Check sheet for the modelled part. Datum: model origin and axes. Units: mm. Face numbers are marked on the shaded views. A direction names the side the tool comes from. Coordinates: 2 decimals unless noted, no trailing zeros. Order: outer loops, then holes, each group sorted by start corner. A loop starts at its lowest first (then second) coordinate and runs counter-clockwise, first axis right, second up. Notation, with made-up numbers: M -1,-20 L 55,-20 A18 ccw 55,-1 Z; hole C -12,28 d8. An arc over 180 degrees is marked long. Answer in a Markdown table with one row per item. Add a question column.
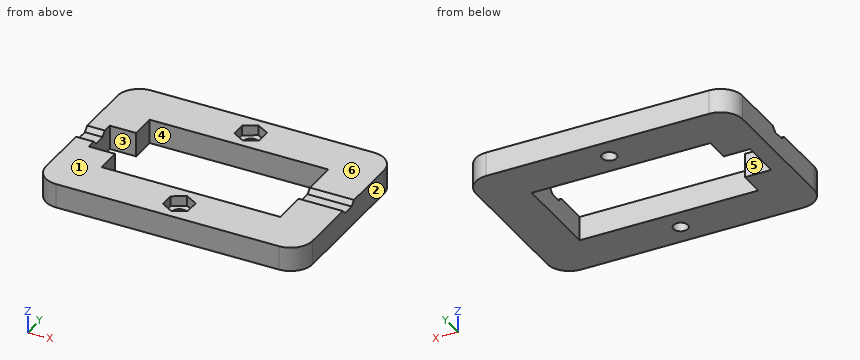
from build123d import *

# Parameters (mm, degrees)
F0_W     = 60.5
F0_H     = 40.5
F0_W_2   = 40.5
F0_H_2   = 20.5
F1_DEPTH = 5.5
F2_W     = 10
F2_H     = 2.8
F3_DEPTH = 1
F4_R     = 1.65
F5_DEPTH = 25
F6_W     = 6
F6_H     = 9
F7_DEPTH = 25
F9_DEPTH = 2.3
F10_SIZE = 0.99999
F11_R    = 5


# Not quite as in the source:
# - a fillet or chamfer is up to 0.001 mm smaller than in the source, because OpenCascade refuses the exact size


with BuildPart() as f1:
    # F0 (on Top) → F1 (new body)
    with BuildSketch(Plane.XY):
        Rectangle(F0_W, F0_H)
        Rectangle(F0_W_2, F0_H_2, mode=Mode.SUBTRACT)
    extrude(amount=F1_DEPTH)

    # F2 (on face) → F3 (cut)
    with BuildSketch(Plane.XY.offset(5.5)):
        with Locations((-25.25, 0)):
            Rectangle(F2_W, F2_H)
        with Locations((25.25, 0)):
            Rectangle(F2_W, F2_H)
    extrude(amount=-F3_DEPTH, mode=Mode.SUBTRACT)

    # F4 (on face) → F5 (cut)
    with BuildSketch(Plane.XY.offset(5.5)):
        with Locations((0, 15.25)):
            Circle(F4_R)
        with Locations((0, -15.25)):
            Circle(F4_R)
    extrude(amount=-F5_DEPTH, mode=Mode.SUBTRACT)

    # F6 (on face) → F7 (cut)
    with BuildSketch(Plane(origin=(0, 0, 0), x_dir=(1, 0, 0), z_dir=(0, 0, -1))):
        with Locations((-23.25, 0)):
            Rectangle(F6_W, F6_H)
    extrude(amount=-F7_DEPTH, mode=Mode.SUBTRACT)

    # F8 (on face) → F9 (cut)
    with BuildSketch(Plane.XY.offset(5.5)):
        Polygon((2.85, 13.6045517328), (2.85, 16.8954482672), (0, 18.5408965344), (-2.85, 16.8954482672), (-2.85, 13.6045517328), (0, 11.9591034656), align=None)
        Polygon((-2.85, -16.8954482672), (0, -18.5408965344), (2.85, -16.8954482672), (2.85, -13.6045517328), (0, -11.9591034656), (-2.85, -13.6045517328), align=None)
    extrude(amount=-F9_DEPTH, mode=Mode.SUBTRACT)

    # F10 (size 1 in the source; OpenCascade refuses exactly that, so slightly less here)
    f10_edges = [f1.edges().sort_by_distance(p)[0] for p in [
        (25.25, 1.4, 5.5),
        (25.25, -1.4, 5.5),
        (-28.25, 1.4, 5.5),
        (-28.25, -1.4, 5.5),
    ]]
    chamfer(f10_edges, length=F10_SIZE)

    # F11
    f11_edges = [f1.edges().sort_by_distance(p)[0] for p in [
        (30.25, 20.25, 2.75),
        (30.25, -20.25, 2.75),
        (-30.25, -20.25, 2.75),
        (-30.25, 20.25, 2.75),
    ]]
    fillet(f11_edges, radius=F11_R)


solid = f1.part
1. Section check A-A on x = 17. Enter the section's corners in (y, z), then the cut area to 3 significant figures.
2. Set-up check for the marked faces 5 and 6: record each of +Z, -Z, +X, -X, +Y, -Y from which the full face is reachable in a straight line by a thin tool's end or side.
3. Scan lines: line 1 (Y direction, x = 0, z = 0.85); line 2 (Y direction, x = -8, z = 3.9); line 3 (X direction, y = -7, z = 4.05). Record each from-to range of solid material in increasing order.
4. Go/stop test with flat-tipped pins: pin 1 Ø0.8 at (x, y) = (25.5, 0) entering from +Z; pin 2 Ø1.7 at (x, y) = (0.5, -16.5) entering from +Z; pin 3 Ø2 at (x, y) = (-29, 0.5) entering from +Z. Record where each tip stops, or that it passes through.
5. Section check C-C on z = 1.3. Enter the section's corners in (x, y), then the cut area to 3 significant figures.
6. Section check B-B on y = 6.5. Enter the section's corners in (x, z).
7. Section check D-D on y = -13. Enter the section's corners in (x, z), then the cut area to 3 significant figures.
8. Release check for a two-part mould opening along X. For the marked faces 1, 2, 3 and 4 record: released by +X, released by -X, zero draft, split by the parting line, or undercut.
Result sheet:
| question | item | result |
|---|---|---|
| 1 | outline | M -20.25,0 L -10.25,0 L -10.25,5.5 L -20.25,5.5 Z; M 10.25,0 L 20.25,0 L 20.25,5.5 L 10.25,5.5 Z |
| 1 | area | 110 mm^2 |
| 2 | face 5 | +Z, -Z |
| 2 | face 6 | +Z, +X, -X, +Y, -Y |
| 3 | line 1 | -20.25 to -16.9, -13.6 to -10.25, 10.25 to 13.6, 16.9 to 20.25 |
| 3 | line 2 | -20.25 to -10.25, 10.25 to 20.25 |
| 3 | line 3 | -30.25 to -20.25, 20.25 to 30.25 |
| 4 | pin 1 | z = 4.5 |
| 4 | pin 2 | z = 3.2 |
| 4 | pin 3 | z = 4.6 |
| 5 | outline | M -30.25,-15.25 A5 ccw -25.25,-20.25 L 25.25,-20.25 A5 ccw 30.25,-15.25 L 30.25,15.25 A5 ccw 25.25,20.25 L -25.25,20.25 A5 ccw -30.25,15.25 Z; hole M -26.25,-4.5 L -20.25,-4.5 L -20.25,-10.25 L 20.25,-10.25 L 20.25,10.25 L -20.25,10.25 L -20.25,4.5 L -26.25,4.5 Z; hole C 0,-15.25 d3.3; hole C 0,15.25 d3.3 |
| 5 | area | 1,530 mm^2 |
| 6 | outline | M -30.25,0 L -20.25,0 L -20.25,5.5 L -30.25,5.5 Z; M 20.25,0 L 30.25,0 L 30.25,5.5 L 20.25,5.5 Z |
| 7 | outline | M -30.25,0 L 30.25,0 L 30.25,5.5 L 1.8,5.5 L 1.8,3.2 L -1.8,3.2 L -1.8,5.5 L -30.25,5.5 Z |
| 7 | area | 324 mm^2 |
| 8 | face 1 | zero draft |
| 8 | face 2 | released by +X |
| 8 | face 3 | undercut |
| 8 | face 4 | undercut |
